```python
from build123d import *

# Parameters (mm, degrees)
F0_W     = 63.5
F0_H     = 114.3
F0_W_2   = 44.45
F0_H_2   = 95.25
F0_W_3   = 19.05
F0_H_3   = 19.05
F1_DEPTH = 44.45
F2_DEPTH = 44.451
F3_DEPTH = 9.525
F4_W     = 44.45
F4_H     = 95.25
F4_W_2   = 19.05
F4_H_2   = 19.05
F5_DEPTH = 9.525


with BuildPart() as f1:
    # F0 (on Front) → F1 (new body)
    with BuildSketch(Plane.XZ):
        with Locations((1.7462493032, -2.8575013936)):
            Rectangle(F0_W, F0_H)
        with Locations((1.7462493032, -2.8575013936)):
            Rectangle(F0_W_2, F0_H_2, mode=Mode.SUBTRACT)
        with Locations((1.7462493032, -2.8575013936)):
            Rectangle(F0_W_2, F0_H_2)
        with Locations((1.7462493032, -31.4325013936)):
            Rectangle(F0_W_3, F0_H_3, mode=Mode.SUBTRACT)
        with Locations((1.7462493032, -2.8575013936)):
            Rectangle(F0_W_3, F0_H_3, mode=Mode.SUBTRACT)
        with Locations((1.7462493032, 25.7174986064)):
            Rectangle(F0_W_3, F0_H_3, mode=Mode.SUBTRACT)
        with Locations((1.7462493032, -31.4325013936)):
            Rectangle(F0_W_3, F0_H_3)
        with Locations((1.7462493032, 25.7174986064)):
            Rectangle(F0_W_3, F0_H_3)
        with Locations((1.7462493032, -2.8575013936)):
            Rectangle(F0_W_3, F0_H_3)
    extrude(amount=F1_DEPTH)

    # F0 (on Front) → F2 (cut, through all)
    with BuildSketch(Plane.XZ):
        with Locations((1.7462493032, 25.7174986064)):
            Rectangle(F0_W_3, F0_H_3)
        with Locations((1.7462493032, -2.8575013936)):
            Rectangle(F0_W_3, F0_H_3)
        with Locations((1.7462493032, -31.4325013936)):
            Rectangle(F0_W_3, F0_H_3)
    extrude(amount=F2_DEPTH, mode=Mode.SUBTRACT)

    # F0 (on Front) → F3 (cut)
    with BuildSketch(Plane.XZ):
        with Locations((1.7462493032, -2.8575013936)):
            Rectangle(F0_W_2, F0_H_2)
        with Locations((1.7462493032, -31.4325013936)):
            Rectangle(F0_W_3, F0_H_3, mode=Mode.SUBTRACT)
        with Locations((1.7462493032, -2.8575013936)):
            Rectangle(F0_W_3, F0_H_3, mode=Mode.SUBTRACT)
        with Locations((1.7462493032, 25.7174986064)):
            Rectangle(F0_W_3, F0_H_3, mode=Mode.SUBTRACT)
    extrude(amount=F3_DEPTH, mode=Mode.SUBTRACT)

    # F4 (on face) → F5 (cut)
    with BuildSketch(Plane.XZ.offset(44.45)):
        with Locations((1.7462493032, -2.8575013936)):
            Rectangle(F4_W, F4_H)
        with Locations((1.7462493032, -31.4325013936)):
            Rectangle(F4_W_2, F4_H_2, mode=Mode.SUBTRACT)
        with Locations((1.7462493032, -2.8575013936)):
            Rectangle(F4_W_2, F4_H_2, mode=Mode.SUBTRACT)
        with Locations((1.7462493032, 25.7174986064)):
            Rectangle(F4_W_2, F4_H_2, mode=Mode.SUBTRACT)
    extrude(amount=-F5_DEPTH, mode=Mode.SUBTRACT)


solid = f1.part
```
Work out the finished part from the listing and answer in its coordinate system (mm). A direction names the side the tool comes from. Give positions to 0.01 mm unless a question says otherwise; leave off trailing zeros. Loops run counter-clockwise (first coordinate to the right, second up) from the corner with the lowest first, then second, coordinate; pieces in that order, holes last. Notation, with made-up numbers: (44.5, -7) -> (50.5, -7) arc R3 ccw to (50.5, -2) -> close; hole circle Ø9 at (19.5, 18.25). An arc over 180 degrees is marked (long way). One line per question, with ' | ' between items. Start each with the question number.
1) Section A-A, the plane z = -30 is taken. Determine the outline of the cut face in (x, y) (3 decimals).
2) Section D-D, the plane y = -4.5 is taken. Determine the outline of the cut face in (x, z).
3) This flat-tipped pin is pushed along its axis until it touches: pin 1 (8 mm diameter, centred on x = -5, z = -23, fed in from +Y) (3 decimals). Where does it stop, or does it pass through?
4) Straight lines are drawn through the part: L1, parallel to Z at x = -9.5, y = -4.5; L2, parallel to X at y = -3, z = 7; L3, parallel to X at y = -19, z = -39. For each, find the intervals that lie inside material, in ascending order.
5) Determine the mould class of faces 4 (the face through (-20.479, -40, -4)), 5 (the face through (-30.004, -22, -4)) for opening direction Z: +Z half, -Z half, draft (parallel to the pull), parting line (faces both ways), or undercut.
6) Section B-B, the plane y = -29 is taken. Determine the outline of the cut face in (x, z), then the cut area to 3 significant figures.
7) For faces 1 (the face through (-8, -34.925, -2)), 2 (the face through (2, -22, 35.242)), 3 (the face through (23.971, -5, -4)), determine the directions among +Z, -Z, +X, -X, +Y, -Y from which every point of the face is accessible in a straight line to the end or side of a thin tool.
Resolved:
1) outline: (-30.004, -44.45) -> (-20.479, -44.45) -> (-20.479, -34.925) -> (-7.779, -34.925) -> (-7.779, -9.525) -> (-20.479, -9.525) -> (-20.479, 0) -> (-30.004, 0) -> close; (11.271, -34.925) -> (23.971, -34.925) -> (23.971, -44.45) -> (33.496, -44.45) -> (33.496, 0) -> (23.971, 0) -> (23.971, -9.525) -> (11.271, -9.525) -> close
2) outline: (-30, -60.01) -> (33.5, -60.01) -> (33.5, 54.29) -> (-30, 54.29) -> close; hole (-20.48, -50.48) -> (23.97, -50.48) -> (23.97, 44.77) -> (-20.48, 44.77) -> close
3) pin 1: y = -9.525
4) L1: -60.01 to -50.48, 44.77 to 54.29 | L2: -30 to -20.48, 23.97 to 33.5 | L3: -30 to -7.78, 11.27 to 33.5
5) face 4: undercut | face 5: draft
6) outline: (-30, -60.01) -> (33.5, -60.01) -> (33.5, 54.29) -> (-30, 54.29) -> close; hole (-7.78, -40.96) -> (11.27, -40.96) -> (11.27, -21.91) -> (-7.78, -21.91) -> close; hole (-7.78, -12.38) -> (11.27, -12.38) -> (11.27, 6.67) -> (-7.78, 6.67) -> close; hole (-7.78, 16.19) -> (11.27, 16.19) -> (11.27, 35.24) -> (-7.78, 35.24) -> close | area: 6,170 mm2
7) face 1: -Y | face 2: +Y, -Y | face 3: +Y
